from build123d import *

# Parameters (mm, degrees)
SKETCH1_R           = 8.15
BOSS_EXTRUDE1_DEPTH = 1.3
SKETCH1_3_R         = 3
BOSS_EXTRUDE2_DEPTH = 0.4
FILLET3_R           = 0.7
FILLET4_R           = 0.5


with BuildPart() as part:
    # Sketch1 → Boss-Extrude1 (new body)
    with BuildSketch(Plane(origin=(0, 0, 0), x_dir=(1, 0, 0), z_dir=(0, 1, 0))):
        with Locations(Location((0, 0, 0), (0, 0, 270))):
            Circle(SKETCH1_R)
        with BuildLine():
            ThreePointArc((-2.75, -3), (-5.75, 0), (-2.75, 3))
            Line((-2.75, 3), (2.75, 3))
            ThreePointArc((2.75, 3), (4.871320344, 2.121320344), (5.75, 0))
            ThreePointArc((5.75, 0), (4.871320344, -2.121320344), (2.75, -3))
            Line((2.75, -3), (-2.75, -3))
        make_face(mode=Mode.SUBTRACT)
    extrude(amount=BOSS_EXTRUDE1_DEPTH)

    # Sketch1_3 → Boss-Extrude2 (add)
    with BuildSketch(Plane(origin=(0, 0, 0), x_dir=(1, 0, 0), z_dir=(0, 1, 0))):
        with Locations((2.75, 0)):
            Circle(SKETCH1_3_R)
        with Locations((-2.75, 0)):
            Circle(SKETCH1_3_R)
        with BuildLine():
            Line((2.75, 3), (-2.75, 3))
            ThreePointArc((-2.75, 3), (-1.106356736, 2.509668668), (0, 1.198957881))
            ThreePointArc((0, 1.198957881), (1.106356736, 2.509668668), (2.75, 3))
        make_face()
        with BuildLine():
            ThreePointArc((0, -1.198957881), (-1.106356736, -2.509668668), (-2.75, -3))
            Line((-2.75, -3), (2.75, -3))
            ThreePointArc((2.75, -3), (1.106356736, -2.509668668), (0, -1.198957881))
        make_face()
    extrude(amount=BOSS_EXTRUDE2_DEPTH)

    # Fillet3
    fillet3_edges = [part.edges().sort_by_distance(p)[0] for p in [
        (0, 1.3, 3),
        (-5.75, 1.3, 0),
        (0, 1.3, -3),
        (5.75, 1.3, 0),
    ]]
    fillet(fillet3_edges, radius=FILLET3_R)

    # Fillet4
    fillet4_edges = [part.edges().sort_by_distance(p)[0] for p in [
        (0, 0, -8.15),
    ]]
    fillet(fillet4_edges, radius=FILLET4_R)


solid = part.part
Here's how the part is built. I have some questions about the finished solid (model axes, mm). Coordinates: 2 decimals unless noted, no trailing zeros. Write each loop counter-clockwise with the first axis right and the second up, starting at its lowest first coordinate (ties: lowest second). Pieces come first, ordered by that corner, then holes.
Item 1: If I drill on line 1 (Z direction, x = 1.5, y = 0.65); line 2 (Z direction, x = 2.5, y = 0.8); line 3 (Y direction, x = 0.75, z = 1.75), over which ranges is the centre line in solid material (lowest first)?
Item 2: I want a section at A-A on y = 1. Write out the boundary of the cut face in (x, z).
Item 3: Will these pins go through, and if not, where does the flat tip stop? pin 1 (3 mm diameter, centred on x = 3.5, z = -1.5, fed in from +Y); pin 2 (1.8 mm diameter, centred on x = 1.5, z = 0, fed in from +Y).
Item 4: If we mould it in two halves opening along Z, with no side actions, what happens to faces 1 (the flat face through (0, 0.4, 0)), 2 (the cylindrical face through (-4.959, 0.894, -6.468)), 3 (the flat face through (0, 1.3, -4))? For each: +Z half, -Z half, draft (parallel to the pull), parting line (faces both ways), or undercut.
Item 5: I want a section at B-B on x = 0. Write out the boundary of the cut face in (y, z), and give its area (3 significant figures).
Findings below:
1. line 1: z = -8.01 to -3, 3 to 8.01
1. line 2: z = -7.76 to -3.03, 3.03 to 7.76
1. line 3: y = 0 to 0.4
2. outline: circle Ø16.3 at (0, 0); hole (-2.75, -3.13) - (2.75, -3.13) arc R3.13 ccw to (2.75, 3.13) - (-2.75, 3.13) arc R3.13 ccw to start
3. pin 1: stops at y = 1.07
3. pin 2: stops at y = 0.4
4. face 1: undercut
4. face 2: parting line
4. face 3: draft
5. outline: (0, -7.65) arc R0.5 ccw to (0.5, -8.15) - (1.3, -8.15) - (1.3, -3.7) arc R0.7 ccw to (0.6, -3) - (0.4, -3) - (0.4, 3) - (0.6, 3) arc R0.7 ccw to (1.3, 3.7) - (1.3, 8.15) - (0.5, 8.15) arc R0.5 ccw to (0, 7.65) - close
5. area: 15.5 mm2
